Could you check a few things on this model? Use its own coordinates, in mm. Face numbers are marked on the shaded views. A direction names the side the tool comes from. Round coordinates to 2 decimals unless told otherwise and drop trailing zeros. Loops run counter-clockwise (first coordinate to the right, second up) from the corner with the lowest first, then second, coordinate; pieces in that order, holes last. Notation, with made-up numbers: (36.5, -33.5) -> (95.5, -33.5) arc R33 ccw to (95.5, 1.5) -> close; hole circle Ø8 at (28.25, 47.5). An arc over 180 degrees is marked (long way). Put each result on its own line as item: value. Start each with the question number.
1. Which directions (+Z, -Z, +X, -X, +Y, -Y) give clear straight access to the entire face, cutting with the end or side of a thin tool? Please do the marked faces 1 and 2.
2. Imagine slicing it at D-D, the plane y = 4.75. Count the separate pieces of the cut face and the enclosed holes in it, and give its area (3 significant figures).
3. Imagine slicing it at A-A, the plane x = -50.5. Please give me the cut outline in (y, z).
4. Imagine slicing it at B-B, the plane y = -2. Please give me the cut outline in (x, z).
5. Imagine slicing it at C-C, the plane z = 1.75. Please give me the cut outline in (x, y) (3 decimals).
6. I need wall thicknesses on line 1 (X direction, y = 1, z = 3); line 2 (X direction, y = -5.5, z = 0.5); line 3 (X direction, y = 4, z = -4.75). Which ranges of each line are inside material? Lowest first, please. Write a range as [from, to].
7. I'm going to push flat-ended pins straight in: P1, Ø3, axis at x = 48, y = -0.5, coming from the +Z side; P2, Ø2, axis at y = 5, z = 4, coming from the -X side; P3, Ø3, axis at y = 3, z = 8, coming from the -X side. Where does each tip first touch, or does it pass through?
```python
from build123d import *

# Parameters (mm, degrees)
F0_W     = 6.35
F0_H     = 12.446
F0_W_2   = 13.208
F0_W_3   = 87.884
F1_DEPTH = 6.35
F2_DEPTH = 12.7
F4_DEPTH = 12.447
F5_R     = 5.08
F6_R     = 3.175
F7_W     = 9.779
F7_H     = 1.778
F8_DEPTH = 12.447


with BuildPart() as f1:
    # F0 (on Top) → F1 (new body)
    with BuildSketch(Plane.XY):
        with Locations((-60.325, 0)):
            Rectangle(F0_W, F0_H)
        with Locations((-50.546, 0)):
            Rectangle(F0_W_2, F0_H)
        Rectangle(F0_W_3, F0_H)
        with Locations((50.546, 0)):
            Rectangle(F0_W_2, F0_H)
        with Locations((60.325, 0)):
            Rectangle(F0_W, F0_H)
    extrude(amount=-F1_DEPTH)

    # F0 (on Top) → F2 (join)
    with BuildSketch(Plane.XY):
        with Locations((-60.325, 0)):
            Rectangle(F0_W, F0_H)
        Rectangle(F0_W_3, F0_H)
        with Locations((60.325, 0)):
            Rectangle(F0_W, F0_H)
    extrude(amount=F2_DEPTH)

    # F3 (on face) → F4 (cut, through all)
    with BuildSketch(Plane.XZ.offset(6.223)):
        with BuildLine():
            ThreePointArc((-57.15, 0.396875), (-57.4306330038, -0.2806330038), (-56.753125, 0))
            Line((-56.753125, 0), (-57.15, 0))
            Line((-57.15, 0), (-57.15, 0.396875))
        make_face()
        with BuildLine():
            Line((-43.942, 0), (-44.338875, 0))
            ThreePointArc((-44.338875, 0), (-43.942, -0.396875), (-43.545125, 0))
            ThreePointArc((-43.545125, 0), (-43.6613669962, 0.2806330038), (-43.942, 0.396875))
            Line((-43.942, 0.396875), (-43.942, 0))
        make_face()
        with BuildLine():
            Line((43.942, 0), (43.942, 0.396875))
            ThreePointArc((43.942, 0.396875), (43.6613669962, -0.2806330038), (44.338875, 0))
            Line((44.338875, 0), (43.942, 0))
        make_face()
        with BuildLine():
            Line((57.15, 0), (56.753125, 0))
            ThreePointArc((56.753125, 0), (57.15, -0.396875), (57.546875, 0))
            ThreePointArc((57.546875, 0), (57.4306330038, 0.2806330038), (57.15, 0.396875))
            Line((57.15, 0.396875), (57.15, 0))
        make_face()
    extrude(amount=-F4_DEPTH, mode=Mode.SUBTRACT)

    # F5
    f5_edges = [f1.edges().sort_by_distance(p)[0] for p in [
        (63.5, 0, 12.7),
        (-63.5, 0, 12.7),
    ]]
    fillet(f5_edges, radius=F5_R)

    # F6
    f6_edges = [f1.edges().sort_by_distance(p)[0] for p in [
        (0, -6.223, 12.7),
        (0, 6.223, 12.7),
        (-63.5, -6.223, 0.635),
        (63.5, -6.223, 0.635),
        (-63.5, 6.223, 0.635),
        (63.5, 6.223, 0.635),
    ]]
    fillet(f6_edges, radius=F6_R)

    # F7 (on face) → F8 (cut, through all)
    with BuildSketch(Plane.XZ.offset(6.223)):
        with Locations((-50.546, -1.68275)):
            Rectangle(F7_W, F7_H)
        with Locations((50.546, -1.68275)):
            Rectangle(F7_W, F7_H)
    extrude(amount=-F8_DEPTH, mode=Mode.SUBTRACT)


solid = f1.part
```
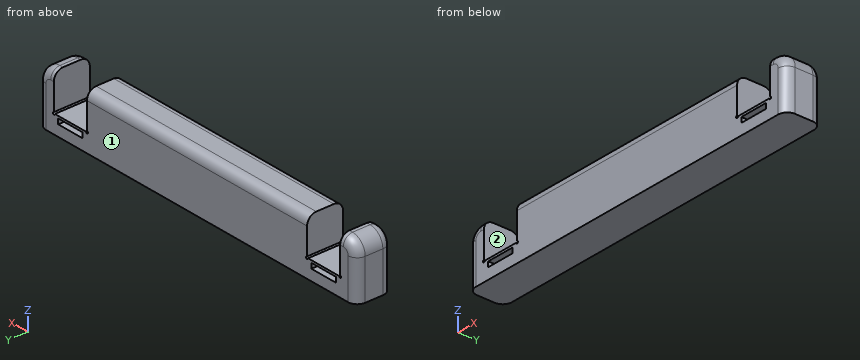
Entries:
1. face 1: +Z, -Z, +X, -X, +Y
1. face 2: +Z, +Y, -Y
2. separate pieces: 1
2. enclosed holes: 2
2. area: 1,970 mm^2
3. outline: (-6.22, -6.35) -> (6.22, -6.35) -> (6.22, -2.57) -> (-6.22, -2.57) -> close; (-6.22, -0.79) -> (6.22, -0.79) -> (6.22, 0) -> (-6.22, 0) -> close
4. outline: (-63.5, -6.35) -> (63.5, -6.35) -> (63.5, 7.62) arc R5.08 ccw to (58.42, 12.7) -> (57.15, 12.7) -> (57.15, 0.4) arc R0.4 cw (long way) to (56.75, 0) -> (44.34, 0) arc R0.4 cw (long way) to (43.94, 0.4) -> (43.94, 12.7) -> (-43.94, 12.7) -> (-43.94, 0.4) arc R0.4 cw (long way) to (-44.34, 0) -> (-56.75, 0) arc R0.4 cw (long way) to (-57.15, 0.4) -> (-57.15, 12.7) -> (-58.42, 12.7) arc R5.08 ccw to (-63.5, 7.62) -> close; hole (-55.44, -2.57) -> (-45.66, -2.57) -> (-45.66, -0.79) -> (-55.44, -0.79) -> close; hole (45.66, -2.57) -> (55.44, -2.57) -> (55.44, -0.79) -> (45.66, -0.79) -> close
5. outline: (-63.5, -3.048) arc R3.175 ccw to (-60.325, -6.223) -> (-57.15, -6.223) -> (-57.15, 6.223) -> (-60.325, 6.223) arc R3.175 ccw to (-63.5, 3.048) -> close; (-43.942, -6.223) -> (43.942, -6.223) -> (43.942, 6.223) -> (-43.942, 6.223) -> close; (57.15, -6.223) -> (60.325, -6.223) arc R3.175 ccw to (63.5, -3.048) -> (63.5, 3.048) arc R3.175 ccw to (60.325, 6.223) -> (57.15, 6.223) -> close
6. line 1: [-63.5, -57.15], [-43.94, 43.94], [57.15, 63.5]
6. line 2: [-62.34, -57.15], [-43.94, 43.94], [57.15, 62.34]
6. line 3: [-63.35, 63.35]
7. P1: z = 0
7. P2: x = -63.35
7. P3: x = -63.5
